CAD build for the part. Positions are in the model's coordinates, mm. A direction names the side the tool comes from. Coordinates: 2 decimals unless noted, no trailing zeros. Order: outer loops, then holes, each group sorted by start corner. A loop starts at its lowest first (then second) coordinate and runs counter-clockwise, first axis right, second up. Notation, with made-up numbers: (44.25, -23.5) - (74.25, -23.5) arc R26 ccw to (74.25, -3.5) - close; hole circle Ø1 at (61.25, 76.25). An arc over 180 degrees is marked (long way). Write each question's results on one line, items separated by ' | '. Start each with the question number.
Q1. Band-saw the part on A-A, the plane y = 1. Write the cut outline in (x, z), then the cut area to 3 significant figures.
Q2. Band-saw the part on B-B, the plane y = 8.25. Write the cut outline in (x, z).
Q3. Band-saw the part on C-C, the plane y = 4.25. Write the cut outline in (x, z).
Q4. Wall check: probe 1 along Z at (x, y) = (-0.25, -0.25); probe 2 along Y at (x, z) = (-4, -7); probe 3 along Y at (x, z) = (7.5, 0.5). Give the ranges that are in metal, low to high.
Q5. Pull direction X, two halves, no side cores. Call faces 4 (the flat face through (6, -8.584, -2)), 5 (the cylindrical face through (-9.76, 3.33, -2.17)), 6 (the conical face through (-0.481, 4.395, 0.924)): released by +X, released by -X, zero draft, split by the parting line, or undercut.
Q6. Which spindle directions (+Z, -Z, +X, -X, +Y, -Y) get a long thin tool onto all of the face, cutting with end or side? Do faces 1 (the cylindrical face through (-7.81, -6.56, -1.73)), 2 (the flat face through (6, 11.416, -2)), 3 (the flat face through (0, 16.416, 0)). Say none if no direction does.
Q7. Band-saw the part on D-D, the plane y = 14.5. Write the cut outline in (x, z).
Q8. Pin check, flat tips, straight feed: P1, Ø1, axis at x = -3, z = 7.5, coming from the +Y side; P2, Ø1, axis at x = 1.5, y = 12.5, coming from the -Z side; P3, Ø3, axis at x = 3.5, y = 1, coming from the +Z side. Stop position of each tip, or through.
```python
from build123d import *

# Parameters (mm, degrees)
SKETCH1_R        = 5
HEAD_DEPTH       = 8
SKETCH3_R        = 4
NECK_DEPTH       = 2
SKETCH6_R        = 3
HEAD_KNOB_DEPTH  = 2.5
HEAD_HOLE_D      = 6
HEAD_HOLE_DEPTH  = 5
HEAD_HOLE_TIP    = 1.802581857
HEAD_ROUNDNESS_R = 1
EADY_INSERT_R    = 0.5
SCALE1_SCALE     = 2


with BuildPart() as part:
    # Sketch1 → Head (new body)
    with BuildSketch(Plane(origin=(0, 0, 0), x_dir=(1, 0, 0), z_dir=(0, 1, 0))):
        with Locations(Location((0, 0, 0), (0, 0, 270))):
            Circle(SKETCH1_R)
    extrude(amount=HEAD_DEPTH)

    # Sketch3 → Neck (add)
    with BuildSketch(Plane(origin=(0, 0, 0), x_dir=(1, 0, 0), z_dir=(0, 1, 0))):
        with Locations(Location((0, 0, 0), (0, 0, 270))):
            Circle(SKETCH3_R)
    extrude(amount=-NECK_DEPTH)

    # Sketch6 → Head knob (add)
    with BuildSketch(Plane(origin=(0, 8, 0), x_dir=(1, 0, 0), z_dir=(0, 1, 0))):
        with Locations(Location((0, 0, 0), (0, 0, 270))):
            Circle(SKETCH6_R)
    extrude(amount=HEAD_KNOB_DEPTH)

    # Head hole
    with Locations(Plane(origin=(0, -2, 0), x_dir=(-1, 0, 0), z_dir=(0, -1, 0))):
        with Locations((0, 0)):
            Hole(HEAD_HOLE_D / 2, depth=HEAD_HOLE_DEPTH)
            with Locations((0, 0, -(HEAD_HOLE_DEPTH + HEAD_HOLE_TIP / 2))):  # 118° drill point
                Cone(0, HEAD_HOLE_D / 2, HEAD_HOLE_TIP, mode=Mode.SUBTRACT)

    # Head roundness
    head_roundness_edges = [part.edges().sort_by_distance(p)[0] for p in [
        (0, 0, -5),
        (0, 8, -5),
    ]]
    fillet(head_roundness_edges, radius=HEAD_ROUNDNESS_R - 0.0001)  # a hair under: the kernel refuses the full size

    # Eady insert
    eady_insert_edges = [part.edges().sort_by_distance(p)[0] for p in [
        (0, 10.5, -3),
    ]]
    fillet(eady_insert_edges, radius=EADY_INSERT_R)


with BuildPart() as part_1:
    # Scale1: scaled about (0, 4.58400844, 0)
    add(part.part.scale(SCALE1_SCALE).moved(Location((0, -4.58400844, 0))))


solid = part_1.part
```
Results below:
1) outline: circle Ø20 at (0, 0); hole circle Ø12 at (0, 0) | area: 201 mm²
2) outline: circle Ø20 at (0, 0)
3) outline: circle Ø20 at (0, 0); hole circle Ø2.57 at (0, 0)
4) probe 1: z = -10 to -5.99, 5.99 to 10 | probe 2: y = -4.58 to 11.42 | probe 3: y = -8.58 to 11.42
5) face 4: zero draft | face 5: split by the parting line | face 6: undercut
6) face 1: -Y | face 2: +Y | face 3: +Z, -Z, +X, -X, +Y
7) outline: circle Ø12 at (0, 0)
8) P1: stops at y = 11.42 | P2: stops at z = -5.92 | P3: stops at z = 9.8
